Geometry check sheet. Reference: drawing and pictorial views, mm from the part's lowest x, y, z. Give positions to 0.01 mm unless a question says otherwise; leave off trailing zeros. Loops run counter-clockwise (first coordinate to the right, second up) from the corner with the lowest first, then second, coordinate; pieces in that order, holes last. Notation, with made-up numbers: M 43,3.25 L 88,3.25 A16 ccw 88,8.25 Z; hole C 81.5,-38 d9. An arc over 180 degrees is marked long. One line per question, with ' | ' between items. Start each with the question number.
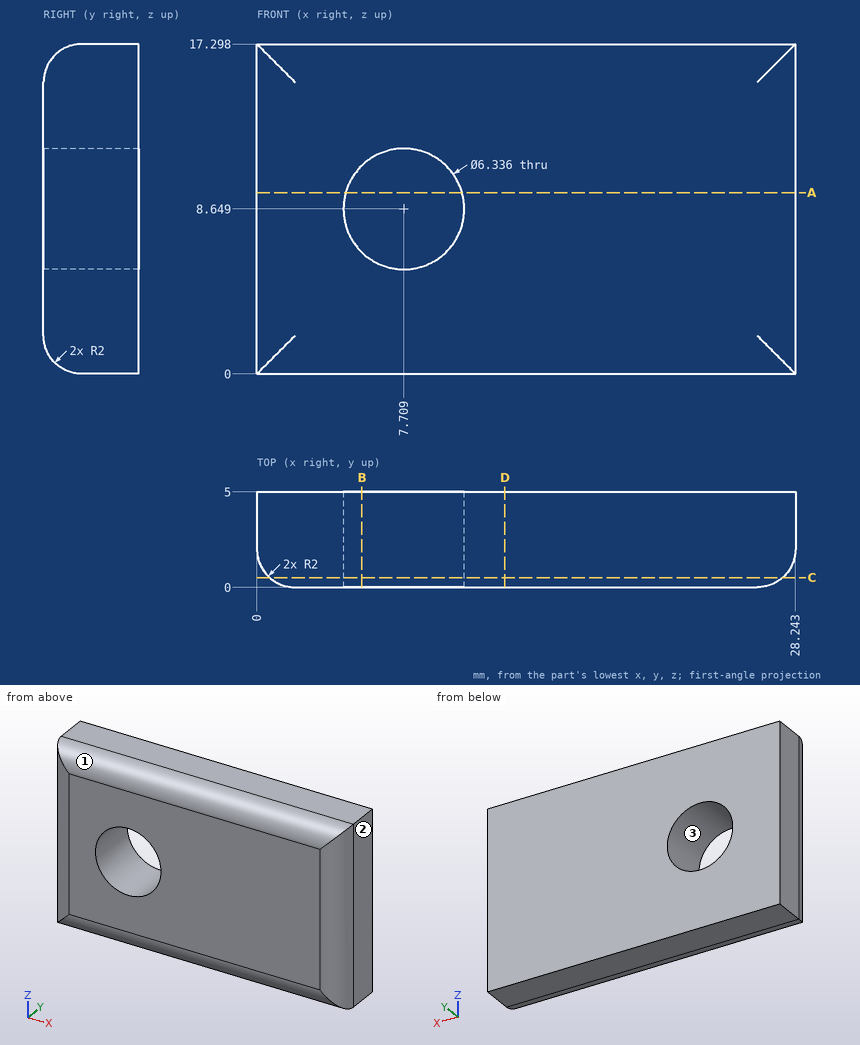
Q1. Draft check along X on the marked faces 1, 2 and 3. Enter one of: released by +X, released by -X, zero draft, split by the parting line, or undercut.
Q2. Cross-section at D-D (x = 13). Record the cut outline in (y, z).
Q3. Cross-section at C-C (y = 0.5). Record the cut outline in (x, z).
Q4. Cross-section at B-B (x = 5.5). Record the cut outline in (y, z).
Q5. Material ranges on probe 1 along Z at (x, y) = (6, 4.6); probe 2 along X at (y, z) = (3.2, 9.25); probe 3 along X at (y, z) = (1.9, 5), recorded low to high. Write a range as from..to.
Q6. Cross-section at A-A (z = 9.5). Record the cut outline in (x, y), and give its area (3 significant figures).
Q7. Depth check by flat-ended pin: P1, Ø4, axis at x = 7.71, z = 8.65, coming from the -Y side; P2, Ø1, axis at x = 22, z = 9, coming from the -Y side. Enter the tip coordinate at first touch or a pass-through.
Solved:
1) face 1: zero draft | face 2: released by +X | face 3: undercut
2) outline: M 0,2 A2 ccw 2,0 L 5,0 L 5,17.3 L 2,17.3 A2 ccw 0,15.3 Z
3) outline: M 0.68,0.68 L 27.57,0.68 L 27.57,16.62 L 0.68,16.62 Z; hole C 7.71,8.65 d6.34
4) outline: M 0,2 A2 ccw 2,0 L 5,0 L 5,6.38 L 0,6.38 Z; M 0,10.92 L 5,10.92 L 5,17.3 L 2,17.3 A2 ccw 0,15.3 Z
5) probe 1: z = 0..5.98, 11.32..17.3 | probe 2: x = 0..4.6, 10.82..28.24 | probe 3: x = 0..28.24
6) outline: M 0,2 A2 ccw 2,0 L 4.66,0 L 4.66,5 L 0,5 Z; M 10.76,0 L 26.24,0 A2 ccw 28.24,2 L 28.24,5 L 10.76,5 Z | area: 109 mm²
7) P1: passes through | P2: stops at y = 0
